Autodesk Inventor part; units mm, degrees
ref_plane "YZ Plane" through (0, 0, 0) normal (1, 0, 0) x (0, 1, 0)
ref_plane "XZ Plane" through (0, 0, 0) normal (0, 1, 0) x (-1, 0, 0)
ref_plane "XY Plane" through (0, 0, 0) normal (0, 0, 1) x (1, 0, 0)
sketch "Sketch1" plane through (0, 0, 0) normal (0, 0, 1) x (1, 0, 0)
  line L0 (0, 277.6336) -> (196.3166, 196.3166) construction
  line L1 (196.3166, 196.3166) -> (277.6336, 0) construction
  line L2 (277.6336, 0) -> (196.3166, -196.3166) construction
  line L3 (196.3166, -196.3166) -> (0, -277.6336) construction
  line L4 (0, -277.6336) -> (-196.3166, -196.3166) construction
  line L5 (-196.3166, -196.3166) -> (-277.6336, 0) construction
  line L6 (-277.6336, 0) -> (-196.3166, 196.3166) construction
  line L7 (-196.3166, 196.3166) -> (0, 277.6336)
  line L8 (-196.3166, 196.3166) -> (0, 277.6336)
  line L9 (-461.2666, 773.8898) -> (-221.0579, 873.3874)
  line L10 (-98.1583, 236.9751) -> (-341.1623, 823.6386) construction
  line L11 (-221.0579, 873.3874) -> (0, 873.3874)
  line L12 (0, 873.3874) -> (0, 277.6336)
  line L13 (-461.2666, 773.8898) -> (-617.5782, 617.5782)
  line L14 (-617.5782, 617.5782) -> (-196.3166, 196.3166)
  point P0 (0, 0)
  point P1 (0, 0)
  dimension "d0" = 513
  dimension "d2" = 260
  dimension "d3" = 635
extrude "Extrusion1" add sketch "Sketch1" along normal mid plane 0.5
sketch "Sketch7" plane through (0, 0, 0.25) normal (0, 0, 1) x (1, 0, 0)
  line L0 (-13, 868.3874) -> (-5, 868.3874)
  line L1 (-5, 868.3874) -> (-5, 860.3874)
  line L2 (-5, 860.3874) -> (-13, 860.3874)
  line L3 (-13, 860.3874) -> (-13, 868.3874)
  line L4 (0, 873.3874) -> (-221.0579, 873.3874)
  line L5 (0, 277.6336) -> (0, 873.3874)
  point P0 (0, 0)
  dimension "d54" = 8
  dimension "d55" = 8
  dimension "d56" = 5
  dimension "d57" = 5
extrude "Extrusion5" [suppressed]
pattern_linear "Rectangular Pattern1" [suppressed]
equation "\"d0\" = Барабан_габарит_по_кассетам"
equation "\"d2\" = Кассета_длина_грани"
equation "\"d3\" = Кассета_высота"
equation "\"BendRadius\" = Thickness"
equation "\"BendReliefWidth\" = Thickness"
equation "\"BendReliefDepth\" = 0.5 * Thickness"
equation "\"CornerReliefSize\" = 4 * Thickness"
equation "\"MinimumRemnant\" = 2 * Thickness"
equation "\"TransitionRadius\" = BendRadius"
equation "\"JacobiRadiusSize\" = BendRadius"
equation "\"GapSize\" = Thickness"
properties part number "ДМФ 01 57 Сетка кассеты v2.0"
Can you work these out from the model? Positions are in its coordinate system, mm. Give positions to 0.01 mm unless a question says otherwise; leave off trailing zeros. Write each loop counter-clockwise with the first axis right and the second up, starting at its lowest first coordinate (ties: lowest second). Pieces come first, ordered by that corner, then holes. Notation, with made-up numbers: (80, -11) -> (84, -11) arc R35 ccw to (84, 23) -> close; hole circle Ø1 at (-34, 4). An arc over 180 degrees is marked (long way). Write item = value, one per line.
(1) Suppose I cut it at C-C on x = -569. Write out the boundary of the cut face in (y, z), then the cut area to 3 significant figures.
Worked out:
outline = (569, -0.25) -> (666.16, -0.25) -> (666.16, 0.25) -> (569, 0.25) -> close
area = 48.6 mm^2
(2) I need wall thicknesses on probe 1 along X at (y, z) = (241.5, -0.05); probe 2 along Y at (x, z) = (-149.5, 0.05); probe 3 along Y at (x, z) = (-185.5, 0.15). Which ranges of each line are inside material? Lowest first, please. Write a range as from..to.
Worked out:
probe_1 = -241.5..-87.23
probe_2 = 215.71..873.39
probe_3 = 200.8..873.39
(3) Suppose I cut it at A-A on y = 472. Write out the boundary of the cut face in (x, z).
Worked out:
outline = (-472, -0.25) -> (0, -0.25) -> (0, 0.25) -> (-472, 0.25) -> close
(4) Suppose I cut it at B-B on z = 0.05. Write out the boundary of the cut face in (x, y).
Worked out:
outline = (-617.58, 617.58) -> (-196.32, 196.32) -> (0, 277.63) -> (0, 873.39) -> (-221.06, 873.39) -> (-461.27, 773.89) -> close
